Build history of the part. All positions in model axes, mm. Round coordinates to 2 decimals unless told otherwise and drop trailing zeros. Order: outer loops, then holes, each group sorted by start corner. A loop starts at its lowest first (then second) coordinate and runs counter-clockwise, first axis right, second up. Notation, with made-up numbers: M 59,-5.75 L 98,-5.75 A19 cw 98,4.25 Z; hole C -5.5,40 d8. An arc over 180 degrees is marked long. One line per item, written item: value. Start each with the question number.
Item 1: Band-saw the part on C-C, the plane z = 16.5. Write the cut outline in (x, y).
Item 2: Probe L1, parallel to X at y = 30, z = 5; L2, parallel to Z at x = 28, y = -0.5; L3, parallel to Z at x = 30.5, y = -9. List the from-to ranges inside material, lowest first.
Item 3: Pin check, flat tips, straight feed: pin 1 (10 mm diameter, centred on x = 13, z = 31, fed in from -Y); pin 2 (5 mm diameter, centred on x = 20.5, z = 38.5, fed in from +Y); pin 3 (3 mm diameter, centred on y = 3, z = 32, fed in from +X). Stop position of each tip, or through.
Solid Edge part; units mm, degrees
sketch "Sketch1" plane through (0, 0, 0) normal (0, 0, 1) x (1, 0, 0)
  line L0 (-56.5685, 0) -> (0, -56.5685)
  line L1 (0, -56.5685) -> (56.5685, 0)
  line L2 (56.5685, 0) -> (0, 56.5685)
  line L3 (0, 56.5685) -> (-56.5685, 0)
extrude "Protrusion1" add sketch "Sketch1" along normal up to vertex (56.5685 mm away)
sketch "Sketch2" plane through (0, 0, 0) normal (0.7071, -0.7071, 0) x (0, 0, -1)
  line L0 (-56.5685, 0) -> (0, -40)
extrude "Cutout1" cut sketch "Sketch2" along normal mid plane 80 material side at (-14.171, -14.171, 28.3131)
pattern_circular "Pattern1" count 4 over 360 about axis through (0, 0, 0) along (0, 0, -1) of "Cutout1"
Output:
1. outline: M -40.07,0 L 0,-40.07 L 40.07,0 L 0,40.07 Z
2. L1: x = -21.57 to 21.57
2. L2: z = 0 to 28.07
2. L3: z = 0 to 17.07
3. pin 1: stops at y = -19.64
3. pin 2: stops at y = 1.1
3. pin 3: stops at x = 23.69
